The listing builds one solid part. Answer for the finished solid, in the listing's coordinates (mm). A direction names the side the tool comes from. Give positions to 0.01 mm unless a question says otherwise; leave off trailing zeros. Order: outer loops, then holes, each group sorted by start corner. A loop starts at its lowest first (then second) coordinate and runs counter-clockwise, first axis right, second up. Notation, with made-up numbers: (-25.75, 40) -> (24.25, 40) arc R12 ccw to (24.25, 52) -> close; hole circle Ø6 at (16, 8.25). An arc over 180 degrees is marked (long way). One line per question, with ' | ' between items. Start each with the question number.
Autodesk Inventor part; units mm, degrees
ref_plane "YZ Plane" through (0, 0, 0) normal (1, 0, 0) x (0, 1, 0)
ref_plane "XZ Plane" through (0, 0, 0) normal (0, 1, 0) x (-1, 0, 0)
ref_plane "XY Plane" through (0, 0, 0) normal (0, 0, 1) x (1, 0, 0)
sketch "Szkic1" plane through (0, 0, 0) normal (0, 1, 0) x (-1, 0, 0)
  line L0 (0, 0) -> (10.5, 0)
  line L1 (10.5, 0) -> (10.5, -15.75)
  line L2 (10.5, -15.75) -> (0, -15.75)
  line L3 (0, -15.75) -> (0, 0)
  line L4 (7.75, -15.75) -> (2.75, -15.75)
  line L5 (2.75, -15.75) -> (2.75, -20.25)
  line L6 (2.75, -20.25) -> (7.75, -20.25)
  line L7 (7.75, -20.25) -> (7.75, -15.75)
  line L8 (7.75, 0) -> (2.75, 0)
  line L9 (2.75, 0) -> (2.75, 4.5)
  line L10 (2.75, 4.5) -> (7.75, 4.5)
  line L11 (7.75, 4.5) -> (7.75, 0)
  circle A0 centre (5.25, 2.25) radius 1.55
  circle A1 centre (5.25, -18) radius 1.55
  point P0 (5.25, -20.25)
  point P1 (7.75, -18)
  point P2 (5.25, 4.5)
  point P3 (7.75, 2.25)
  dimension "d0" = 10.5
  dimension "d1" = 15.75
  dimension "d2" = 5
  dimension "d3" = 4.5
  dimension "d4" = 2.75
  dimension "d5" = 5
  dimension "d6" = 4.5
  dimension "d7" = 2.75
  dimension "d8" = 3.1
  dimension "d9" = 3.1
  dimension "d10" = 2.25
  dimension "d11" = 2.5
  dimension "d12" = 2.25
  dimension "d13" = 2.5
extrude "Wyciągnięcie proste1" add sketch "Szkic1" along normal blind 1
fillet "Zaokrąglenie1" radius 2.5 4 edges at (-2.75, 0.5, 4.5) (-7.75, 0.5, 4.5) (-2.75, 0.5, -20.25) (-7.75, 0.5, -20.25)
properties part number "1XV2"
(1) Given P1, Ø0.5, axis at y = 0.5, z = -17, coming from the -X side, flat-ended and moving along its own axis, determine where the tip first touches the part or whether it passes through.
(2) Consider line 1 (Z direction, x = -5.25, y = 0.75); line 2 (Z direction, x = -6.25, y = 0.5); line 3 (X direction, y = 0.2, z = -17.75). Determine where each line is inside the solid, lowest interval first.
(3) The part is cut by section C-C on x = -6. Determine the outline of the cut face in (y, z), plus the area to 3 significant figures.
(4) The part is cut by section A-A on y = 0.5. State how many separate pieces and enclosed holes the cut face has, plus the area to 3 significant figures.
(5) The part is cut by section D-D on x = -9.5. Determine the outline of the cut face in (y, z), plus the area to 4 significant figures.
(6) The part is cut by section B-B on z = 2.25. Determine the outline of the cut face in (x, y), plus the area to 3 significant figures.
(7) Determine the mould class of faces 4 (the face through (-10.5, 0.5, -7.8)), 5 (the face through (-5.048, 0.493, -19.537)), 6 (the face through (-3.502, 0.507, 3.787)), 7 (the face through (-5, 1, -8)) for opening direction X: pulls with the +X half, pulls with the -X half, needs draft (parallel to the pull), parting line crosses it, or undercut.
(8) For faces 1 (the face through (-2.75, 0.5, 1)), 2 (the face through (-1.4, 0.5, -15.75)), 3 (the face through (-7.75, 0.5, 1)), determine the directions among +Z, -Z, +X, -X, +Y, -Y from which every point of the face is accessible in a straight line to the end or side of a thin tool.
Result sheet:
1) P1: stops at x = -7.75
2) line 1: z = -20.25 to -19.55, -16.45 to 0.7, 3.8 to 4.5 | line 2: z = -20.04 to -19.18, -16.82 to 1.07, 3.43 to 4.29 | line 3: x = -7.75 to -6.78, -3.72 to -2.75
3) outline: (0, -20.13) -> (1, -20.13) -> (1, -19.36) -> (0, -19.36) -> close; (0, -16.64) -> (1, -16.64) -> (1, 0.89) -> (0, 0.89) -> close; (0, 3.61) -> (1, 3.61) -> (1, 4.38) -> (0, 4.38) -> close | area: 19.1 mm^2
4) separate pieces: 1 | enclosed holes: 2 | area: 190 mm^2
5) outline: (0, -15.75) -> (1, -15.75) -> (1, 0) -> (0, 0) -> close | area: 15.75 mm^2
6) outline: (-7.74, 0) -> (-6.8, 0) -> (-6.8, 1) -> (-7.74, 1) -> close; (-3.7, 0) -> (-2.76, 0) -> (-2.76, 1) -> (-3.7, 1) -> close | area: 1.88 mm^2
7) face 4: pulls with the -X half | face 5: undercut | face 6: pulls with the +X half | face 7: needs draft
8) face 1: +Z, +X, +Y, -Y | face 2: -Z, +X, +Y, -Y | face 3: +Z, -X, +Y, -Y
